Build history of the part. All positions in model axes, mm. Face numbers are marked on the shaded views. A direction names the side the tool comes from. Give positions to 0.01 mm unless a question says otherwise; leave off trailing zeros. Order: outer loops, then holes, each group sorted by start corner. A loop starts at its lowest first (then second) coordinate and runs counter-clockwise, first axis right, second up. Notation, with made-up numbers: M 51,55 L 66,55 A22 cw 66,79 Z; hole C -0.5,52.25 d4. An arc over 180 degrees is marked long. One line per item, written item: value.
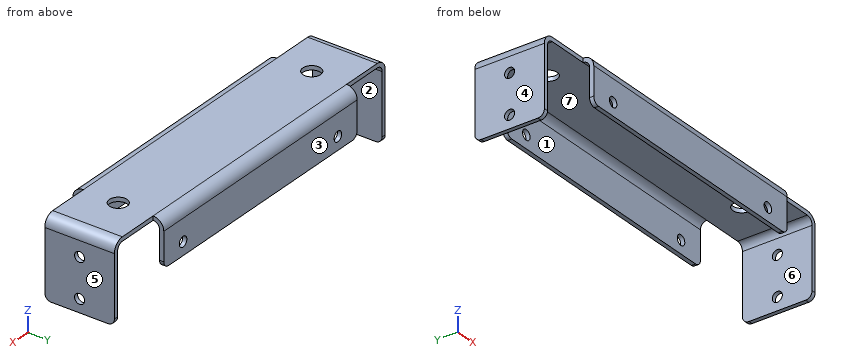
from build123d import *

# Parameters (mm, degrees)
BASE_FLANGE1_DEPTH           = 127
SKETCH6_W                    = 2.032
SKETCH6_H                    = 34.036
BOSS_EXTRUDE1_DEPTH          = 25.4
EDGE_FLANGE1_STRIP_W         = 14.478
EDGE_FLANGE1_STRIP_H         = 2.032
EDGE_FLANGE1_STRIP_CUT_DEPTH = 34.036
EDGE_FLANGE1_DEPTH           = 34.036
SKETCH10_R                   = 2.4511
CUT_EXTRUDE1_DEPTH           = 188.190417757
SKETCH11_R                   = 2.4511
CUT_EXTRUDE2_DEPTH           = 164.257993679
SKETCH12_R                   = 4.3688
CUT_EXTRUDE3_DEPTH           = 164.257993679
FILLET1_R                    = 3.175


# Sheet-metal steps are written as plain solids
with BuildPart() as part:
    # Sketch1 → Base-Flange1 (new body)
    with BuildSketch(Plane(origin=(0, 0, 0), x_dir=(0, 0, -1), z_dir=(1, 0, 0))):
        with BuildLine():
            Line((22.225, 0), (5.207, 0))
            ThreePointArc((5.207, 0), (1.52509499, 1.52509499), (0, 5.207))
            Line((0, 5.207), (0, 39.243))
            ThreePointArc((0, 39.243), (1.52509499, 42.92490501), (5.207, 44.45))
            Line((5.207, 44.45), (22.225, 44.45))
            Line((22.225, 44.45), (22.225, 42.418))
            Line((22.225, 42.418), (5.207, 42.418))
            ThreePointArc((5.207, 42.418), (2.96193597, 41.48806403), (2.032, 39.243))
            Line((2.032, 39.243), (2.032, 5.207))
            ThreePointArc((2.032, 5.207), (2.96193597, 2.96193597), (5.207, 2.032))
            Line((5.207, 2.032), (22.225, 2.032))
            Line((22.225, 2.032), (22.225, 0))
        make_face()
    extrude(amount=BASE_FLANGE1_DEPTH)

    # Sketch6 → Boss-Extrude1 (add)
    with BuildSketch(Plane(origin=(127, 0, 0), x_dir=(0, 0, -1), z_dir=(1, 0, 0))):
        with Locations((1.016, 22.225)):
            Rectangle(SKETCH6_W, SKETCH6_H)
    boss_extrude1 = extrude(amount=BOSS_EXTRUDE1_DEPTH)

    # Edge-Flange1 strip (across the edge) → Edge-Flange1 strip cut (cut)
    with BuildSketch(Plane(origin=(152.4, 39.243, -2.032), x_dir=(-1, 0, 0), z_dir=(0, -1, 0))):
        with Locations((-2.032, -1.016)):
            Rectangle(EDGE_FLANGE1_STRIP_W, EDGE_FLANGE1_STRIP_H)
    edge_flange1_strip_cut = extrude(amount=EDGE_FLANGE1_STRIP_CUT_DEPTH, mode=Mode.SUBTRACT)

    # Edge-Flange1 section (across the edge) → Edge-Flange1 (add)
    with BuildSketch(Plane(origin=(152.4, 39.243, -2.032), x_dir=(-1, 0, 0), z_dir=(0, -1, 0))):
        with BuildLine():
            Line((0, 3.175), (0, 36.068))
            Line((0, 36.068), (2.032, 36.068))
            Line((2.032, 36.068), (2.032, 3.175))
            ThreePointArc((2.032, 3.175), (2.96193597, 0.92993597), (5.207, 0))
            Line((5.207, 0), (5.207, -2.032))
            ThreePointArc((5.207, -2.032), (1.52509499, -0.50690501), (0, 3.175))
        make_face()
    edge_flange1 = extrude(amount=EDGE_FLANGE1_DEPTH)

    # Mirror1: Boss-Extrude1, Edge-Flange1 strip cut, Edge-Flange1 across plane
    add(boss_extrude1.mirror(Plane(origin=(63.5, 0, 0), x_dir=(0, 0, 1), z_dir=(1, 0, 0))))
    add(edge_flange1_strip_cut.mirror(Plane(origin=(63.5, 0, 0), x_dir=(0, 0, 1), z_dir=(1, 0, 0))), mode=Mode.SUBTRACT)
    add(edge_flange1.mirror(Plane(origin=(63.5, 0, 0), x_dir=(0, 0, 1), z_dir=(1, 0, 0))))

    # Sketch10 → Cut-Extrude1 (cut, through all)
    with BuildSketch(Plane(origin=(152.4, 0, 0), x_dir=(0, 0, -1), z_dir=(1, 0, 0))):
        with Locations((12.7, 22.225)):
            Circle(SKETCH10_R)
        with Locations((31.75, 22.225)):
            Circle(SKETCH10_R)
    extrude(amount=-CUT_EXTRUDE1_DEPTH, mode=Mode.SUBTRACT)

    # Sketch11 → Cut-Extrude2 (cut, through all)
    with BuildSketch(Plane(origin=(0, 44.45, 0), x_dir=(1, 0, 0), z_dir=(0, 1, 0))):
        with Locations(Location((12.7, 15.875, 0), (0, 0, 270))):
            Circle(SKETCH11_R)
        with Locations(Location((114.3, 15.875, 0), (0, 0, 270))):
            Circle(SKETCH11_R)
    extrude(amount=-CUT_EXTRUDE2_DEPTH, mode=Mode.SUBTRACT)

    # Sketch12 → Cut-Extrude3 (cut, through all)
    with BuildSketch(Plane.XY):
        with Locations((0, 22.225)):
            Circle(SKETCH12_R)
        with Locations((127, 22.225)):
            Circle(SKETCH12_R)
    extrude(amount=-CUT_EXTRUDE3_DEPTH, mode=Mode.SUBTRACT)

    # Fillet1
    fillet1_edges = [part.edges().sort_by_distance(p)[0] for p in [
        (-24.384, 5.207, -38.1),
        (0, 1.016, -22.225),
        (-24.384, 39.243, -38.1),
        (0, 43.434, -22.225),
        (127, 1.016, -22.225),
        (151.384, 39.243, -38.1),
        (151.384, 5.207, -38.1),
        (127, 43.434, -22.225),
    ]]
    fillet(fillet1_edges, radius=FILLET1_R)


solid = part.part
1) Tool access for the marked faces 1, 2 and 3: list every direction of +Z, -Z, +X, -X, +Y, -Y with a clear straight run to the whole face (end or side of a thin tool).
Check values:
face 1: -Z, +X, -X
face 2: -Z, +Y, -Y
face 3: +Z, -Z, +X, -X, +Y
2) Saw through at D-D, the plane y = 29. Write the cut outline in (x, z) (3 decimals).
Check values:
outline: M -25.4,-38.1 L -23.368,-38.1 L -23.368,-5.207 A3.175 cw -20.193,-2.032 L 147.193,-2.032 A3.175 cw 150.368,-5.207 L 150.368,-38.1 L 152.4,-38.1 L 152.4,-5.207 A5.207 ccw 147.193,0 L -20.193,0 A5.207 ccw -25.4,-5.207 Z
3) Saw through at A-A, the plane x = 114.3. Write the cut outline in (y, z) (3 decimals), then the cut area to 3 significant figures.
Check values:
outline: M 0,-22.225 L 2.032,-22.225 L 2.032,-18.326 L 0,-18.326 Z; M 0,-13.424 L 2.032,-13.424 L 2.032,-5.207 A3.175 cw 5.207,-2.032 L 39.243,-2.032 A3.175 cw 42.418,-5.207 L 42.418,-13.424 L 44.45,-13.424 L 44.45,-5.207 A5.207 ccw 39.243,0 L 5.207,0 A5.207 ccw 0,-5.207 Z; M 42.418,-22.225 L 44.45,-22.225 L 44.45,-18.326 L 42.418,-18.326 Z
area: 145 mm^2
4) Pin check, flat tips, straight feed: pin 1 (2 mm diameter, centred on x = 74.5, y = 0.5, fed in from -Z) (3 decimals); pin 2 (5 mm diameter, centred on x = 8, y = 14.5, fed in from -Z). Stop position of each tip, or through.
Check values:
pin 1: z = -22.225
pin 2: z = -2.03
5) Mould opens along X. For the marked faces 4, 5, 6 and 7 say: released by +X, released by -X, zero draft, split by the parting line, or undercut.
Check values:
face 4: released by -X
face 5: released by +X
face 6: undercut
face 7: undercut
6) Saw through at C-C, the plane x = 64. Write the cut outline in (y, z) (3 decimals).
Check values:
outline: M 0,-22.225 L 2.032,-22.225 L 2.032,-5.207 A3.175 cw 5.207,-2.032 L 39.243,-2.032 A3.175 cw 42.418,-5.207 L 42.418,-22.225 L 44.45,-22.225 L 44.45,-5.207 A5.207 ccw 39.243,0 L 5.207,0 A5.207 ccw 0,-5.207 Z
7) Saw through at B-B, the plane z = -26. Write the cut outline in (x, y), then the cut area to 3 significant figures.
Check values:
outline: M -25.4,5.21 L -23.37,5.21 L -23.37,39.24 L -25.4,39.24 Z; M 150.37,5.21 L 152.4,5.21 L 152.4,39.24 L 150.37,39.24 Z
area: 138 mm^2
8) Drill centre lines: probe 1 along Y at (x, z) = (103.5, -12); probe 2 along X at (y, z) = (29.5, -20.5); probe 3 along Y at (x, z) = (-23.8, -12.7). Where is each one in solid material? Low to high. Write a range as from..to.
Check values:
probe 1: 0..2.03, 42.42..44.45
probe 2: -25.4..-23.37, 150.37..152.4
probe 3: 5.21..19.77, 24.68..39.24
